Geometry check sheet. Reference: the model listing, model coordinates, mm. A direction names the side the tool comes from. Round coordinates to 2 decimals unless told otherwise and drop trailing zeros. Order: outer loops, then holes, each group sorted by start corner. A loop starts at its lowest first (then second) coordinate and runs counter-clockwise, first axis right, second up. Notation, with made-up numbers: (4, 5) -> (49, 5) arc R25 ccw to (49, 21) -> close; hole circle Ø9 at (-23, 65). An arc over 180 degrees is marked (long way). Use a Markdown table: item, result. Add a question column.
Item 1: Sectioned sample at C-C, the plane y = 19.5. Record the cut outline in (x, z) (3 decimals).
Item 2: Material ranges on probe 1 along Z at (x, y) = (-14, -4.5); probe 2 along Y at (x, z) = (1.5, 25); probe 3 along Y at (x, z) = (0.5, 20.5), recorded low to high. Write a range as [from, to].
Item 3: Sectioned sample at B-B, the plane y = 10. Record the cut outline in (x, z) (3 decimals).
Item 4: Sectioned sample at A-A, the plane x = 0. Record the cut outline in (y, z).
Item 5: Set-up check for faces 1 (the flat face through (15.875, 0, 9)), 2 (the cylindrical face through (-0.413, 23.464, 25.311)): record each of +Z, -Z, +X, -X, +Y, -Y from which the full face is reachable in a straight line by a thin tool's end or side.
Item 6: Sectioned sample at D-D, the plane z = 26. Record the cut outline in (x, y) (3 decimals).
from build123d import *

# Parameters (mm, degrees)
SKETCH1_W           = 31.75
SKETCH1_H           = 63.5
BOSS_EXTRUDE1_DEPTH = 19.05
SKETCH2_R           = 3.175
BOSS_EXTRUDE2_DEPTH = 12.7


with BuildPart() as part:
    # Sketch1 → Boss-Extrude1 (new body)
    with BuildSketch(Plane.XY):
        Rectangle(SKETCH1_W, SKETCH1_H)
    extrude(amount=BOSS_EXTRUDE1_DEPTH)

    # Sketch2 → Boss-Extrude2 (add)
    with BuildSketch(Plane.XY.offset(19.05)):
        with Locations((0, 20.315619897)):
            Circle(SKETCH2_R)
    extrude(amount=BOSS_EXTRUDE2_DEPTH)


solid = part.part
Found:
| question | item | result |
|---|---|---|
| 1 | outline | (-15.875, 0) -> (15.875, 0) -> (15.875, 19.05) -> (3.068, 19.05) -> (3.068, 31.75) -> (-3.068, 31.75) -> (-3.068, 19.05) -> (-15.875, 19.05) -> close |
| 2 | probe 1 | z = [0, 19.05] |
| 2 | probe 2 | y = [17.52, 23.11] |
| 2 | probe 3 | y = [17.18, 23.45] |
| 3 | outline | (-15.875, 0) -> (15.875, 0) -> (15.875, 19.05) -> (-15.875, 19.05) -> close |
| 4 | outline | (-31.75, 0) -> (31.75, 0) -> (31.75, 19.05) -> (23.49, 19.05) -> (23.49, 31.75) -> (17.14, 31.75) -> (17.14, 19.05) -> (-31.75, 19.05) -> close |
| 5 | face 1 | +Z, -Z, +X, +Y, -Y |
| 5 | face 2 | +Z |
| 6 | outline | circle Ø6.35 at (0, 20.316) |
